```python
from build123d import *

# Parameters (mm, degrees)
ESBO_O1_W                = 350
ESBO_O1_H                = 180
ESBO_O1_R                = 2
ESBO_O1_R_2              = 15
ESBO_O1_R_3              = 4
ESBO_O1_R_4              = 1.65
ESBO_O1_W_2              = 20
ESBO_O1_H_2              = 20
RESSALTO_EXTRUS_O1_DEPTH = 6
ESBO_O2_R                = 2
CORTE_EXTRUS_O1_DEPTH    = 10
ESBO_O3_R                = 2
CORTE_EXTRUS_O2_DEPTH    = 10
ESBO_O4_R                = 1.55
CORTE_EXTRUS_O3_DEPTH    = 10


with BuildPart() as part:
    # Esboço1 → Ressalto-extrusão1 (new body)
    with BuildSketch(Plane.XY):
        Rectangle(ESBO_O1_W, ESBO_O1_H)
        with Locations((-132.5, -56.5)):
            Circle(ESBO_O1_R, mode=Mode.SUBTRACT)
        with Locations((-67.5, -56.5)):
            Circle(ESBO_O1_R, mode=Mode.SUBTRACT)
        with Locations((-100, -64)):
            Circle(ESBO_O1_R_2, mode=Mode.SUBTRACT)
        with Locations((-60, -64)):
            Circle(ESBO_O1_R_3, mode=Mode.SUBTRACT)
        with Locations((-140, -64)):
            Circle(ESBO_O1_R_3, mode=Mode.SUBTRACT)
        with Locations((-67.5, -71.5)):
            Circle(ESBO_O1_R, mode=Mode.SUBTRACT)
        with Locations((-132.5, -71.5)):
            Circle(ESBO_O1_R, mode=Mode.SUBTRACT)
        with Locations((10, -3)):
            Circle(ESBO_O1_R_4, mode=Mode.SUBTRACT)
        with Locations((10, -28)):
            Circle(ESBO_O1_R_4, mode=Mode.SUBTRACT)
        with Locations((-155, 60)):
            Circle(ESBO_O1_R_4, mode=Mode.SUBTRACT)
        with Locations((-45, 60)):
            Circle(ESBO_O1_R_4, mode=Mode.SUBTRACT)
        with Locations((-45, 5)):
            Circle(ESBO_O1_R_4, mode=Mode.SUBTRACT)
        with Locations((-155, 5)):
            Circle(ESBO_O1_R_4, mode=Mode.SUBTRACT)
        with Locations((75, -51.75)):
            Rectangle(ESBO_O1_W_2, ESBO_O1_H_2, mode=Mode.SUBTRACT)
    extrude(amount=RESSALTO_EXTRUS_O1_DEPTH)

    # Esboço2 → Corte-extrusão1 (cut)
    with BuildSketch(Plane.XY.offset(6)):
        with Locations((-165, 80)):
            Circle(ESBO_O2_R)
        with Locations((165, 80)):
            Circle(ESBO_O2_R)
        with Locations((165, -80)):
            Circle(ESBO_O2_R)
        with Locations((-165, -80)):
            Circle(ESBO_O2_R)
    extrude(amount=-CORTE_EXTRUS_O1_DEPTH, mode=Mode.SUBTRACT)

    # Esboço3 → Corte-extrusão2 (cut)
    with BuildSketch(Plane.XY.offset(6)):
        with Locations((80, -67.5)):
            Circle(ESBO_O3_R)
        with Locations((80, -36.5)):
            Circle(ESBO_O3_R)
        with Locations((70, -36.5)):
            Circle(ESBO_O3_R)
        with Locations((70, -67.5)):
            Circle(ESBO_O3_R)
    extrude(amount=-CORTE_EXTRUS_O2_DEPTH, mode=Mode.SUBTRACT)

    # Esboço4 → Corte-extrusão3 (cut)
    with BuildSketch(Plane.XY.offset(6)):
        with Locations((112.5, 75)):
            Circle(ESBO_O4_R)
        with Locations((137.5, 75)):
            Circle(ESBO_O4_R)
        with Locations((12.5, 75)):
            Circle(ESBO_O4_R)
        with Locations((37.5, 75)):
            Circle(ESBO_O4_R)
        with Locations((137.5, -75)):
            Circle(ESBO_O4_R)
        with Locations((112.5, -75)):
            Circle(ESBO_O4_R)
        with Locations((12.5, -75)):
            Circle(ESBO_O4_R)
        with Locations((37.5, -75)):
            Circle(ESBO_O4_R)
    extrude(amount=-CORTE_EXTRUS_O3_DEPTH, mode=Mode.SUBTRACT)


solid = part.part
```
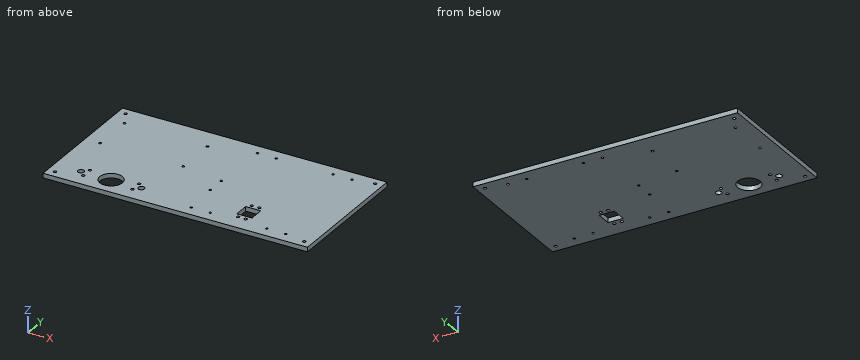
Geometry: final body of the model. Coordinates: model frame, mm. Give positions to 0.01 mm unless a question says otherwise; leave off trailing zeros. Write each loop counter-clockwise with the first axis right and the second up, starting at its lowest first coordinate (ties: lowest second). Pieces come first, ordered by that corner, then holes.
1. Pin query (flat end, axial travel): P1, Ø2, axis at x = -45, y = 5, coming from the +Z side. Return the tip coordinate at first contact, or that it passes through.
2. Section query A-A, the plane x = -60. Return loops of the section in (y, z), then the cut area to 3 significant figures.
3. Line query: probe 1 along X at (y, z) = (-45.5, 2.1); probe 2 along Y at (x, z) = (-67.5, 4.6); probe 3 along Y at (x, z) = (112.5, 2.6). Output: solid intervals per line, ascending.
4. Section query B-B, the plane z = 1.35. Count the separate pieces of the cut face and the enclosed holes in it, then the cut area to 3 significant figures.
Computed:
1. P1: passes through
2. outline: (-90, 0) - (-68, 0) - (-68, 6) - (-90, 6) - close; (-60, 0) - (90, 0) - (90, 6) - (-60, 6) - close
2. area: 1,030 mm2
3. probe 1: x = -175 to 65, 85 to 175
3. probe 2: y = -90 to -73.5, -69.5 to -58.5, -54.5 to 90
3. probe 3: y = -90 to -76.55, -73.45 to 73.45, 76.55 to 90
4. separate pieces: 1
4. enclosed holes: 30
4. area: 61,500 mm2
